The listing builds one solid part. Answer for the finished solid, in the listing's coordinates (mm). A direction names the side the tool comes from. Coordinates: 2 decimals unless noted, no trailing zeros. Order: outer loops, then holes, each group sorted by start corner. A loop starts at its lowest first (then second) coordinate and runs counter-clockwise, first axis right, second up. Notation, with made-up numbers: (63.25, 4.5) - (87.25, 4.5) arc R20 cw to (87.25, 36.5) - close; hole circle Ø6 at (87.25, -10). An arc over 180 degrees is marked (long way). Use a Markdown table: item, result. Add a question column.
Item 1: A flat-ended cylindrical pin translates along its axis: P1, Ø1.8, axis at x = -7.9, y = 37.68, coming from the -Z side. Find the tip coordinate at first contact, or state that the pin passes through.
Item 2: For faces 4 (the flat face through (-29.37, 59.47, 0.99)), 5 (the flat face through (-18, 60, 2)), determine the directions among +Z, -Z, +X, -X, +Y, -Y from which every point of the face is accessible in a straight line to the end or side of a thin tool.
Item 3: The part is cut by section C-C, the plane z = 1.25. State how many separate pieces and enclosed holes the cut face has, then the cut area to 3 significant figures.
Item 4: Find the intervals of material crossed by line 1 along X through (y, z) = (99, 0.55); line 2 along Y through (x, z) = (-28, 0.15); line 3 along X through (y, z) = (106, 0.45), in increasing order.
Item 5: The part is cut by section A-A, the plane x = -86. Give the vertices of the cut face in (y, z), then the cut area to 3 significant figures.
Item 6: The part is cut by section B-B, the plane y = 150. Give the vertices of the cut face in (x, z), then the cut area to 3 significant figures.
Item 7: The mould has two halves that part along X. Classify faces 1 (the flat face through (-18, 60, 0)), 2 (the flat face through (-31.095, 55.82, 0.986)), 3 (the cylindrical face through (-65.77, 5.36, 0.99)): released by +X, released by -X, zero draft, split by the parting line, or undercut.
from build123d import *

# Parameters (mm, degrees)
SKETCH_1_R      = 1.52
SKETCH_1_R_2    = 1.519999991
SKETCH_1_R_3    = 1.520000009
SKETCH_1_R_4    = 1.520000002
SKETCH_1_R_5    = 3.6
SKETCH_1_R_6    = 1.517381685
SKETCH_1_R_7    = 1.519999997
EXTRUDE_1_DEPTH = 2
FILLET_1_R      = 5


with BuildPart() as part:
    # 草图1 → 凸台-拉伸1 (new body)
    with BuildSketch(Plane.XY):
        with BuildLine():
            ThreePointArc((71.75669201, 78.511901277), (31.878575622, 152.307394815), (-51.703250679, 159.386755327))
            ThreePointArc((-51.703250679, 159.386755327), (-57.956662012, 105.693394177), (-104.68190817, 78.511901277))
            ThreePointArc((-104.68190817, 78.511901277), (-64.803791783, 4.716407738), (18.778034519, -2.362952773))
            ThreePointArc((18.778034519, -2.362952773), (25.031445851, 51.330408377), (71.75669201, 78.511901277))
        make_face()
        with Locations((-94.974509357, 62.049293197)):
            Circle(SKETCH_1_R, mode=Mode.SUBTRACT)
        Circle(SKETCH_1_R, mode=Mode.SUBTRACT)
        with Locations((-32.925216161, 157.023802554)):
            Circle(SKETCH_1_R, mode=Mode.SUBTRACT)
        with Locations((62.049293197, 94.974509357)):
            Circle(SKETCH_1_R, mode=Mode.SUBTRACT)
        with Locations((-47.487254679, 31.024646598)):
            Circle(SKETCH_1_R_2, mode=Mode.SUBTRACT)
        with Locations((-22.372181549, 14.61632244)):
            Circle(SKETCH_1_R_3, mode=Mode.SUBTRACT)
        with Locations((-72.602327809, 47.432970756)):
            Circle(SKETCH_1_R_3, mode=Mode.SUBTRACT)
        with BuildLine():
            ThreePointArc((-12.190085291, 30.286229165), (-11.613016331, 27.517295901), (-14.381949595, 26.940226942))
            Line((-14.381949595, 26.940226942), (-64.57198293, 59.818191506))
            ThreePointArc((-64.57198293, 59.818191506), (-65.149051889, 62.587124769), (-62.380118626, 63.164193728))
            Line((-62.380118626, 63.164193728), (-12.190085291, 30.286229165))
        make_face(mode=Mode.SUBTRACT)
        with Locations((-57.293948747, 69.950264788)):
            Circle(SKETCH_1_R_4, mode=Mode.SUBTRACT)
        with BuildLine():
            ThreePointArc((-12.40781803, 48.360410386), (-11.830749071, 45.591477123), (-14.599682334, 45.014408164))
            Line((-14.599682334, 45.014408164), (-48.059704557, 66.933051206))
            ThreePointArc((-48.059704557, 66.933051206), (-48.636773516, 69.70198447), (-45.867840253, 70.279053429))
            Line((-45.867840253, 70.279053429), (-12.40781803, 48.360410386))
        make_face(mode=Mode.SUBTRACT)
        with BuildLine():
            ThreePointArc((-9.979365756, 61.005797168), (-9.402296797, 58.236863905), (-12.17123006, 57.659794946))
            Line((-12.17123006, 57.659794946), (-37.266246728, 74.098777228))
            ThreePointArc((-37.266246728, 74.098777228), (-37.843315687, 76.867710491), (-35.074382424, 77.44477945))
            Line((-35.074382424, 77.44477945), (-9.979365756, 61.005797168))
        make_face(mode=Mode.SUBTRACT)
        with Locations((-7.900971591, 37.68056061)):
            Circle(SKETCH_1_R, mode=Mode.SUBTRACT)
        with Locations((-25.024244569, 119.343241944)):
            Circle(SKETCH_1_R, mode=Mode.SUBTRACT)
        with Locations((-16.46260808, 78.511901277)):
            Circle(SKETCH_1_R_5, mode=Mode.SUBTRACT)
        with BuildLine():
            Line((-20.727239862, 99.346486961), (4.367776805, 82.907504679))
            ThreePointArc((4.367776805, 82.907504679), (4.944845764, 80.138571416), (2.175912501, 79.561502457))
            Line((2.175912501, 79.561502457), (-22.919104167, 96.000484738))
            ThreePointArc((-22.919104167, 96.000484738), (-23.496173126, 98.769418002), (-20.727239862, 99.346486961))
        make_face(mode=Mode.SUBTRACT)
        with BuildLine():
            Line((-18.469699209, 112.103832748), (14.990323014, 90.185189705))
            ThreePointArc((14.990323014, 90.185189705), (15.567391973, 87.416256442), (12.79845871, 86.839187483))
            Line((12.79845871, 86.839187483), (-20.661563513, 108.757830525))
            ThreePointArc((-20.661563513, 108.757830525), (-21.238632472, 111.526763789), (-18.469699209, 112.103832748))
        make_face(mode=Mode.SUBTRACT)
        with Locations((24.368732586, 87.073537766)):
            Circle(SKETCH_1_R_6, mode=Mode.SUBTRACT)
        with BuildLine():
            Line((-18.543266566, 130.083575612), (31.646766769, 97.205611048))
            ThreePointArc((31.646766769, 97.205611048), (32.223835728, 94.436677785), (29.454902465, 93.859608826))
            Line((29.454902465, 93.859608826), (-20.73513087, 126.737573389))
            ThreePointArc((-20.73513087, 126.737573389), (-21.312199829, 129.506506653), (-18.543266566, 130.083575612))
        make_face(mode=Mode.SUBTRACT)
        with Locations((39.677111648, 109.590831797)):
            Circle(SKETCH_1_R_3, mode=Mode.SUBTRACT)
        with Locations((-10.553034612, 142.407480114)):
            Circle(SKETCH_1_R_3, mode=Mode.SUBTRACT)
        with Locations((14.562038518, 125.999155956)):
            Circle(SKETCH_1_R_7, mode=Mode.SUBTRACT)
    extrude(amount=EXTRUDE_1_DEPTH)

    # 圆角1
    fillet_1_edges = [part.edges().sort_by_distance(p)[0] for p in [
        (71.75669201, 78.511901277, 1),
        (18.778034519, -2.362952773, 1),
        (-104.68190817, 78.511901277, 1),
        (-51.703250679, 159.386755327, 1),
    ]]
    fillet(fillet_1_edges, radius=FILLET_1_R)


solid = part.part
Solution:
| question | item | result |
|---|---|---|
| 1 | P1 | passes through |
| 2 | face 4 | +Z, -Z |
| 2 | face 5 | +Z, +X, -X, +Y, -Y |
| 3 | separate pieces | 1 |
| 3 | enclosed holes | 21 |
| 3 | area | 18,000 mm2 |
| 4 | line 1 | x = -63.04 to -23.32, -20.2 to -5.77, 1.53 to 21.61, 28.91 to 69.34 |
| 4 | line 2 | y = -8.95 to 35.86, 40.64 to 53.79, 58.57 to 68.03, 72.81 to 165.97 |
| 4 | line 3 | x = -57.76 to -16.45, -9.15 to 10.92, 18.22 to 67.36 |
| 5 | outline | (24.22, 0) - (82.73, 0) - (82.73, 2) - (24.22, 2) - close |
| 5 | area | 117 mm2 |
| 6 | outline | (-49.13, 0) - (35.23, 0) - (35.23, 2) - (-49.13, 2) - close |
| 6 | area | 169 mm2 |
| 7 | face 1 | zero draft |
| 7 | face 2 | undercut |
| 7 | face 3 | split by the parting line |
